from build123d import *

# Parameters (mm, degrees)
BOSS_EXTRUDE1_DEPTH      = 150
BOSS_EXTRUDE1_DEPTH_BACK = 110
SKETCH1_R                = 25
SKETCH1_R_2              = 14
BOSS_EXTRUDE2_DEPTH      = 30
SKETCH4_R                = 6
CUT_EXTRUDE1_DEPTH       = 30
CUT_EXTRUDE3_DEPTH       = 30
CUT_EXTRUDE4_DEPTH       = 30
BOSS_EXTRUDE3_DEPTH      = 50
BOSS_EXTRUDE3_DEPTH_BACK = 10
SKETCH10_R               = 6
CUT_EXTRUDE5_DEPTH       = 20


with BuildPart() as part:
    # Sketch1 → Boss-Extrude1 (new, two sides: drawn at the far end of the back side and taken through both)
    with BuildSketch(Plane(origin=(0, 0, 0), x_dir=(1, 0, 0), z_dir=(0, 1, 0)).offset(-BOSS_EXTRUDE1_DEPTH_BACK)):
        with Locations(Location((0, 0, 0), (0, 0, 270))):
            Circle(SKETCH1_R)
        with Locations(Location((0, 0, 0), (0, 0, 270))):
            Circle(SKETCH1_R_2, mode=Mode.SUBTRACT)
    extrude(amount=BOSS_EXTRUDE1_DEPTH + BOSS_EXTRUDE1_DEPTH_BACK)

    # Sketch2 → Boss-Extrude2 (add)
    with BuildSketch(Plane(origin=(0, 150, 0), x_dir=(1, 0, 0), z_dir=(0, 1, 0))):
        with BuildLine():
            Line((-23.915836384, 14.561345064), (-21.353425342, 13.00120095))
            ThreePointArc((-21.353425342, 13.00120095), (9.671523715, 23.053451564), (24.237934753, -6.125562743))
            Line((24.237934753, -6.125562743), (43.683817295, -14.479533157))
            Line((43.683817295, -14.479533157), (44.867972274, -11.723126622))
            Line((44.867972274, -11.723126622), (27.66288952, -4.331806018))
            ThreePointArc((27.66288952, -4.331806018), (11.097692173, 25.70683233), (-22.124313852, 17.161431659))
            Line((-22.124313852, 17.161431659), (-39.224178944, 24.402944888))
            Line((-39.224178944, 24.402944888), (-40.408333923, 21.646538353))
            Line((-40.408333923, 21.646538353), (-23.915836384, 14.561345064))
        make_face()
        with BuildLine():
            Line((-43.500856668, 14.266360747), (-24.222080563, 6.187957111))
            ThreePointArc((-24.222080563, 6.187957111), (-9.661815141, -23.057522161), (21.397729285, -12.928154604))
            Line((21.397729285, -12.928154604), (40.848787327, -21.078749702))
            Line((40.848787327, -21.078749702), (39.664632347, -23.835156237))
            Line((39.664632347, -23.835156237), (22.614348516, -16.510337404))
            ThreePointArc((22.614348516, -16.510337404), (-10.742271175, -25.857370516), (-27.656212868, 4.374230197))
            Line((-27.656212868, 4.374230197), (-44.660274485, 11.499458088))
            Line((-44.660274485, 11.499458088), (-43.500856668, 14.266360747))
        make_face()
    extrude(amount=-BOSS_EXTRUDE2_DEPTH)

    # Sketch4 → Cut-Extrude1 (cut)
    with BuildSketch(Plane(origin=(2.798049006, 0, -6.607218549), x_dir=(-0.9208327997677669, 0, -0.38995763214977075), z_dir=(0.3899576321497707, 0, -0.9208327997677668))):
        with Locations(Location((36.350025121, 135, 0), (0, 0, 180))):
            Circle(SKETCH4_R)
    extrude(amount=-CUT_EXTRUDE1_DEPTH, mode=Mode.SUBTRACT)

    # Sketch6 → Cut-Extrude3 (cut)
    with BuildSketch(Plane(origin=(-2.464398676, 0, 5.736482753), x_dir=(0.9188021782605189, 0, 0.39471832643509935), z_dir=(-0.39471832643509935, 0, 0.9188021782605189))):
        Polygon((36.573584503, 150), (45.852123581, 140.721460922), (66.07138883, 154.845920949), align=None)
        Polygon((36.573584503, 120), (62.874627202, 146.301042699), (73.132170225, 136.043499677), (73.132170225, 101.712575759), align=None)
    extrude(amount=-CUT_EXTRUDE3_DEPTH, mode=Mode.SUBTRACT)

    # Sketch7 → Cut-Extrude4 (cut)
    with BuildSketch(Plane(origin=(-2.571593456, 0, 6.137001406), x_dir=(0.9223008864267629, 0, 0.3864726056221933), z_dir=(-0.3864726056221933, 0, 0.9223008864267629))):
        Polygon((-36.416153031, 150), (-45.634436276, 140.781716754), (-52.238797728, 153.982696948), (-36.416153031, 153.982696948), align=None)
        Polygon((-36.416153031, 120), (-66.089359291, 149.67320626), (-66.089359291, 112.136229403), align=None)
    extrude(amount=-CUT_EXTRUDE4_DEPTH, mode=Mode.SUBTRACT)

    # Sketch8 → Boss-Extrude3 (add, two sides: drawn at the far end of the back side and taken through both)
    with BuildSketch(Plane.XZ.offset(110).offset(-BOSS_EXTRUDE3_DEPTH_BACK)):
        with BuildLine():
            Line((-23.915836384, -14.561345064), (-31.938215406, -18.007767043))
            Line((-31.938215406, -18.007767043), (-40.408333923, -21.646538353))
            Line((-40.408333923, -21.646538353), (-39.224178944, -24.402944888))
            Line((-39.224178944, -24.402944888), (-30.760365079, -20.818658126))
            Line((-30.760365079, -20.818658126), (-22.124313852, -17.161431659))
            ThreePointArc((-22.124313852, -17.161431659), (11.097692173, -25.70683233), (27.66288952, 4.331806018))
            Line((27.66288952, 4.331806018), (36.342830359, 8.060717205))
            Line((36.342830359, 8.060717205), (35.15867538, 10.81712374))
            Line((35.15867538, 10.81712374), (24.237934753, 6.125562743))
            ThreePointArc((24.237934753, 6.125562743), (9.671523715, -23.053451564), (-21.353425342, -13.00120095))
            Line((-21.353425342, -13.00120095), (-23.915836384, -14.561345064))
        make_face()
        with BuildLine():
            Line((-27.656212868, -4.374230197), (-36.158243676, -7.936844143))
            Line((-36.158243676, -7.936844143), (-44.660274485, -11.499458088))
            Line((-44.660274485, -11.499458088), (-43.500856668, -14.266360747))
            Line((-43.500856668, -14.266360747), (-34.998825859, -10.703746802))
            Line((-34.998825859, -10.703746802), (-24.222080563, -6.187957111))
            ThreePointArc((-24.222080563, -6.187957111), (-9.661815141, 23.057522161), (21.397729285, 12.928154604))
            Line((21.397729285, 12.928154604), (32.290839196, 17.492704669))
            Line((32.290839196, 17.492704669), (31.139490432, 20.17274682))
            Line((31.139490432, 20.17274682), (22.614348516, 16.510337404))
            ThreePointArc((22.614348516, 16.510337404), (-10.742271175, 25.857370516), (-27.656212868, -4.374230197))
        make_face()
    extrude(amount=BOSS_EXTRUDE3_DEPTH + BOSS_EXTRUDE3_DEPTH_BACK)

    # Sketch10 → Cut-Extrude5 (cut)
    with BuildSketch(Plane(origin=(2.798049006, 0, -6.607218549), x_dir=(-0.9208327997677666, 0, -0.3899576321497714), z_dir=(0.3899576321497714, 0, -0.9208327997677666))):
        with Locations(Location((35.51571532, -149.915667196, 0), (0, 0, 180))):
            Circle(SKETCH10_R)
    extrude(amount=-CUT_EXTRUDE5_DEPTH, mode=Mode.SUBTRACT)


solid = part.part
Model file for the job. Use its own axes, mm. A direction names the side the tool comes from. Coordinates: 2 decimals unless noted, no trailing zeros. Order: outer loops, then holes, each group sorted by start corner. A loop starts at its lowest first (then second) coordinate and runs counter-clockwise, first axis right, second up. Notation, with made-up numbers: M 78,82.5 L 127,82.5 A28 ccw 127,120.5 Z; hole C -37.5,70 d7. An arc over 180 degrees is marked long. Return JSON: item names as keys, results as strings.
1. Flat gauge pins, fed straight in: pin 1 (10 mm diameter, centred on y = -84, z = 14.5, fed in from -X); pin 2 (5 mm diameter, centred on y = -53, z = -15.5, fed in from -X); pin 3 (3 mm diameter, centred on y = 113, z = -15, fed in from +X). Where does each tip first touch, or does it go through?
Ans:
{"pin 1": "x = -23.12", "pin 2": "x = -21.35", "pin 3": "x = 21.04"}
2. Saw through at C-C (x = 0). Give the cut face in (y, z).
Ans:
{"outline": "M -160,-28 L -100,-28 L -100,-25 L 120,-25 L 120,-28 L 150,-28 L 150,-14 L -110,-14 L -110,-25 L -160,-25 Z; M -160,25 L -110,25 L -110,14 L 150,14 L 150,28 L 120,28 L 120,25 L -100,25 L -100,28 L -160,28 Z"}
3. Saw through at D-D (y = 83). Give the cut face in (x, z), and give its area (3 significant figures).
Ans:
{"outline": "C 0,0 d50; hole C 0,0 d28", "area": "1,350 mm^2"}
4. Pull direction Y, two halves, no side cores. Call faces 6 (the face through (-24.855, 135.21, -18.318)), 7 (the face through (-35.478, -155.865, -9.302)), 8 (the face through (39.945, 124.574, 11.264)), 9 (the face through (-6.8, 120, 24.3)): +Y half, -Y half, draft (parallel to the pull), parting line (faces both ways), or undercut.
Ans:
{"face 6": "draft", "face 7": "undercut", "face 8": "-Y half", "face 9": "undercut"}
5. Drill centre lines: probe 1 along Z at (x, y) = (-0.5, -28) (3 decimals); probe 2 along X at (y, z) = (-8, 0); probe 3 along Y at (x, z) = (-33, -19). Where is each one in solid material? Low to high.
Ans:
{"probe 1": "-24.995 to -13.991, 13.991 to 24.995", "probe 2": "-25 to -14, 14 to 25", "probe 3": "-160 to -155.47, -144.37 to -100, 121.36 to 129.18, 140.82 to 148.64"}
6. Saw through at B-B (z = 0). Give the cut face in (x, y).
Ans:
{"outline": "M -28,-160 L -25,-160 L -25,-110 L -14,-110 L -14,150 L -28,150 L -28,120 L -25,120 L -25,-100 L -28,-100 Z; M 14,-110 L 25,-110 L 25,-160 L 28,-160 L 28,-100 L 25,-100 L 25,120 L 28,120 L 28,150 L 14,150 Z"}
7. Saw through at A-A (y = -114.5). Give the cut face in (x, z).
Ans:
{"outline": "M -44.66,-11.5 L -43.5,-14.27 L -24.22,-6.19 A25 cw 21.4,12.93 L 32.29,17.49 L 31.14,20.17 L 22.61,16.51 A28 ccw -27.66,-4.37 Z; M -40.41,-21.65 L -39.22,-24.4 L -22.12,-17.16 A28 ccw 27.66,4.33 L 36.34,8.06 L 35.16,10.82 L 24.24,6.13 A25 cw -21.35,-13 L -23.92,-14.56 Z"}
8. Tool access for faces 1 (the face through (26.94, -129.58, 18.37)), 2 (the face through (-9.58, -10.71, 23.09)), 3 (the face through (10.128, -134.65, -22.856)), 4 (the face through (35.926, 145.426, 20.619)), 5 (the face through (-7, 150, -13)): list every direction of +Z, -Z, +X, -X, +Y, -Y with a clear straight run to the whole face (end or side of a thin tool).
Ans:
{"face 1": "+Z, +Y, -Y", "face 2": "none", "face 3": "-Y", "face 4": "+Z, +X, +Y", "face 5": "+Z, -Z, +X, -X, +Y"}
